Part print with two shaded views. Sizes in mm from the minimum x, y, z corner. A direction names the side the tool comes from. Coordinates: 2 decimals unless noted, no trailing zeros. Write each loop counter-clockwise with the first axis right and the second up, starting at its lowest first coordinate (ties: lowest second). Pieces come first, ordered by that corner, then holes. Notation, with made-up numbers: (63, 62) - (82, 62) arc R28 ccw to (82, 92) - close; hole circle Ø5 at (-4, -24). An arc over 180 degrees is marked (long way). Answer in a Markdown table with one row per item. Add a question column.
Q1. 3-axis set-ups, long thin cutter, end or side, ignore diameter. For the marked faces 1, 2 and 3: which of +Z, -Z, +X, -X, +Y, -Y reach the whole face in a straight line?
Q2. Band-saw the part on A-A (x = 10). List the corners of the cut face in (y, z).
Q3. Band-saw the part on B-B (z = 6.5). State how many separate pieces and enclosed holes the cut face has, and give its area (3 significant figures).
Q4. Drill centre lines: line 1 along X through (y, z) = (4.25, 6.5); line 2 along Z through (x, y) = (16.5, 13.25); line 3 along X through (y, z) = (16.5, 3). Where is each one in solid material? Low to high. Write a range as from..to.
Q5. Band-saw the part on D-D (x = 18.5). List the corners of the cut face in (y, z).
Q6. Band-saw the part on C-C (y = 15.5). List the corners of the cut face in (x, z).
Q7. Pin check, flat tips, straight feed: pin 1 (0.8 mm diameter, centred on y = 20, z = 1, fed in from +X); pin 2 (6 mm diameter, centred on x = 10, y = 15.5, fed in from -Z); pin 3 (2.5 mm diameter, centred on x = 5.32, y = 4.75, fed in from -Z); pin 4 (8 mm diameter, centred on x = 10, y = 15.5, fed in from +Z). Stop position of each tip, or through.
Q8. Two-plate mould, pull along Y, no slides. Class the marked faces 4, 5 and 6: +Y half, -Y half, draft (parallel to the pull), parting line (faces both ways), or undercut.
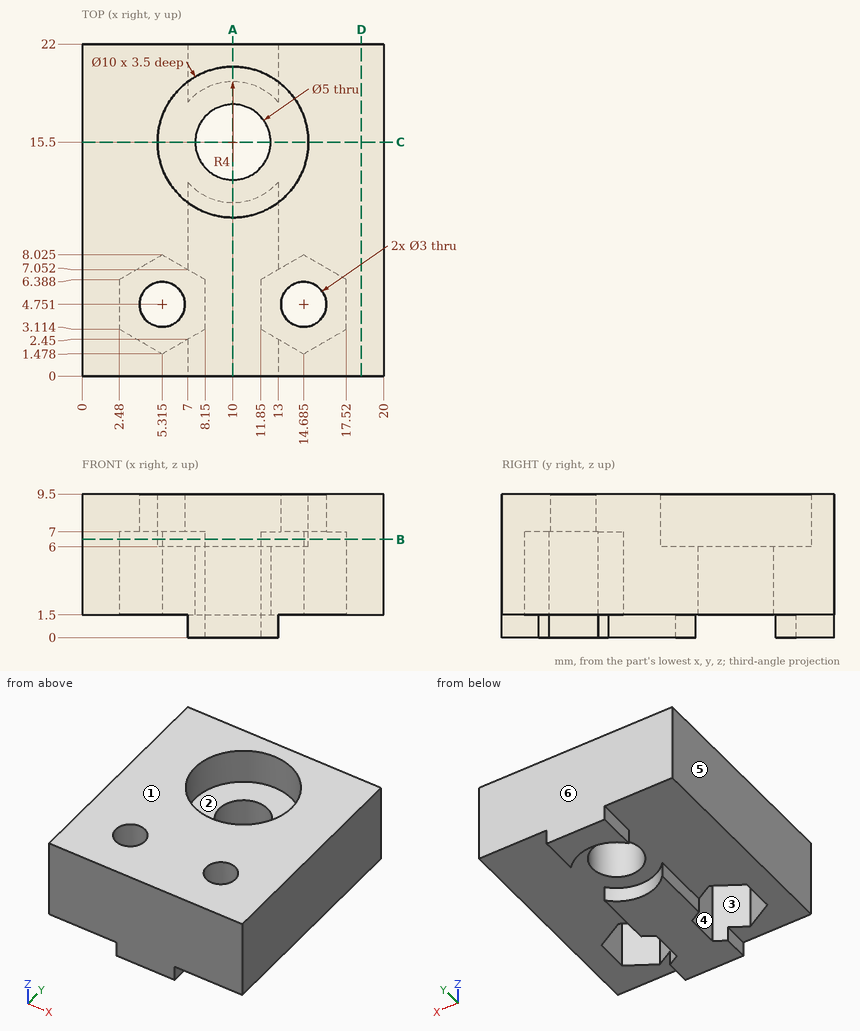
Checked values:
| question | item | result |
|---|---|---|
| 1 | face 1 | +Z, +X, -X, +Y, -Y |
| 1 | face 2 | +Z |
| 1 | face 3 | -Z |
| 2 | outline | (0, 0) - (11.5, 0) - (11.5, 1.5) - (13, 1.5) - (13, 6) - (10.5, 6) - (10.5, 9.5) - (0, 9.5) - close; (18, 1.5) - (19.5, 1.5) - (19.5, 0) - (22, 0) - (22, 9.5) - (20.5, 9.5) - (20.5, 6) - (18, 6) - close |
| 3 | separate pieces | 1 |
| 3 | enclosed holes | 3 |
| 3 | area | 306 mm² |
| 4 | line 1 | x = 0..2.48, 8.15..11.85, 17.52..20 |
| 4 | line 2 | z = 1.5..9.5 |
| 4 | line 3 | x = 0..7.71, 12.29..20 |
| 5 | outline | (0, 1.5) - (22, 1.5) - (22, 9.5) - (0, 9.5) - close |
| 6 | outline | (0, 1.5) - (7.5, 1.5) - (7.5, 6) - (5, 6) - (5, 9.5) - (0, 9.5) - close; (12.5, 1.5) - (20, 1.5) - (20, 9.5) - (15, 9.5) - (15, 6) - (12.5, 6) - close |
| 7 | pin 1 | stops at x = 13 |
| 7 | pin 2 | stops at z = 1.5 |
| 7 | pin 3 | passes through |
| 7 | pin 4 | stops at z = 6 |
| 8 | face 4 | undercut |
| 8 | face 5 | draft |
| 8 | face 6 | +Y half |
